from build123d import *

# Parameters (mm, degrees)
SKETCH1_R           = 34
SKETCH1_R_2         = 1.5
SKETCH1_R_3         = 6.8
SKETCH1_R_4         = 3.5
SKETCH1_W           = 3
SKETCH1_H           = 5
BOSS_EXTRUDE1_DEPTH = 5


with BuildPart() as part:
    # Sketch1 → Boss-Extrude1 (new body)
    with BuildSketch(Plane.XY):
        Circle(SKETCH1_R)
        with Locations((30, 0)):
            Circle(SKETCH1_R_2, mode=Mode.SUBTRACT)
        with Locations((-7.5, -12.990381057)):
            Circle(SKETCH1_R_2, mode=Mode.SUBTRACT)
        with Locations((-7.5, 12.990381057)):
            Circle(SKETCH1_R_2, mode=Mode.SUBTRACT)
        Circle(SKETCH1_R_3, mode=Mode.SUBTRACT)
        with Locations((-17.5, 20)):
            Circle(SKETCH1_R_4, mode=Mode.SUBTRACT)
        with Locations(Location((17.5, 20, 0), (0, 0, 180))):
            Circle(SKETCH1_R_4, mode=Mode.SUBTRACT)
        with Locations(Location((-17.5, -20, 0), (0, 0, 180))):
            Circle(SKETCH1_R_4, mode=Mode.SUBTRACT)
        with Locations((17.5, -20)):
            Circle(SKETCH1_R_4, mode=Mode.SUBTRACT)
        with Locations((20.845079102, 9.72022002)):
            Circle(SKETCH1_R_2, mode=Mode.SUBTRACT)
        with Locations((-20.845079102, 9.72022002)):
            Circle(SKETCH1_R_2, mode=Mode.SUBTRACT)
        with Locations((0, -23)):
            Circle(SKETCH1_R_2, mode=Mode.SUBTRACT)
        Polygon((15.679612774, 8.966590392), (11.148073839, 6.853499083), (12.415928624, 4.134575722), (16.947467559, 6.247667031), align=None, mode=Mode.SUBTRACT)
        Polygon((24.742690644, 13.192773009), (29.27422958, 15.305864318), (30.542084365, 12.586940957), (26.01054543, 10.473849648), align=None, mode=Mode.SUBTRACT)
        Polygon((-16.947467559, 6.247667031), (-12.415928624, 4.134575722), (-11.148073839, 6.853499083), (-15.679612774, 8.966590392), align=None, mode=Mode.SUBTRACT)
        Polygon((-26.01054543, 10.473849648), (-30.542084365, 12.586940957), (-29.27422958, 15.305864318), (-24.742690644, 13.192773009), align=None, mode=Mode.SUBTRACT)
        with Locations((0, -30.5)):
            Rectangle(SKETCH1_W, SKETCH1_H, mode=Mode.SUBTRACT)
        with Locations((0, -15.5)):
            Rectangle(SKETCH1_W, SKETCH1_H, mode=Mode.SUBTRACT)
    extrude(amount=BOSS_EXTRUDE1_DEPTH)


solid = part.part
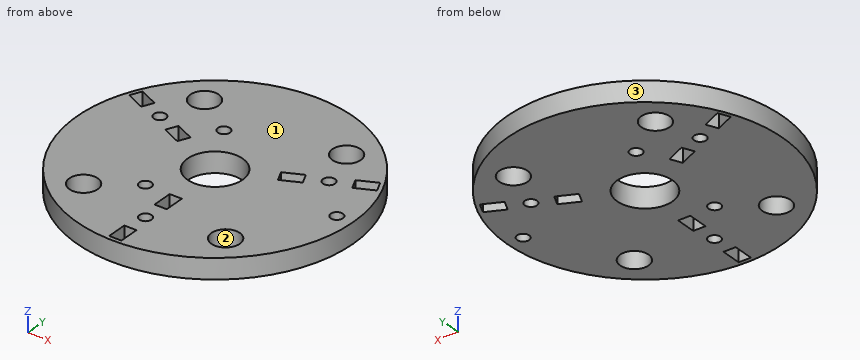
Source: CAD feature listing. Evaluate the final solid. Frame: model axes, mm. Face numbers are marked on the shaded views. Give positions to 0.01 mm unless a question says otherwise; leave off trailing zeros. Write each loop counter-clockwise with the first axis right and the second up, starting at its lowest first coordinate (ties: lowest second). Pieces come first, ordered by that corner, then holes. Notation, with made-up numbers: (-8, 19) -> (41, 19) arc R28 ccw to (41, 46) -> close; hole circle Ø1 at (65, 58). An arc over 180 degrees is marked (long way). Return JSON: item names as keys, results as strings. Group by question number.
1. Mould query, pull axis Y, two halves, no side actions, for the marked faces 1, 2 and 3. Classes: +Y half, -Y half, draft (parallel to the pull), parting line (faces both ways), or undercut.
2. Section D-D, the plane z = 3.85. Count the separate pieces of the cut face and the enclosed holes in it, then the cut area to 3 significant figures.
3. Section C-C, the plane x = 18.5. Output: boundary loops of the cut face in (y, z), then the cut area to 3 significant figures.
4. Section A-A, the plane x = 0. Output: boundary loops of the cut face in (y, z), then the cut area to 3 significant figures.
5. Material intervals for line 1 (X direction, y = 19, z = 2.75); line 2 (Y direction, x = -17.5, z = 1.7); line 3 (Y direction, x = -17, z = 1.2), sorted ascending. Write a range as from..to.
6. Section B-B, the plane y = -20. Output: boundary loops of the cut face in (x, z).
7. Pin query (flat end, axial travel): pin 1 Ø2.5 at (x, y) = (0, -23) entering from +Z; pin 2 Ø1 at (x, z) = (16.5, 4) entering from -Y; pin 3 Ø2.5 at (x, z) = (0.5, 2.5) entering from +Y; pin 4 Ø1 at (x, z) = (6, 4.5) entering from +Y. Return the tip coordinate at first contact, or that it passes through.
Determined:
{
 "1": {"face 1": "draft", "face 2": "undercut", "face 3": "parting line"},
 "2": {"separate pieces": "1", "enclosed holes": "17", "area": "3,200 mm2"},
 "3": {"outline": "(-28.53, 0) -> (-23.35, 0) -> (-23.35, 5) -> (-28.53, 5) -> close; (-16.65, 0) -> (16.65, 0) -> (16.65, 5) -> (-16.65, 5) -> close; (23.35, 0) -> (28.53, 0) -> (28.53, 5) -> (23.35, 5) -> close", "area": "218 mm2"},
 "4": {"outline": "(-34, 0) -> (-33, 0) -> (-33, 5) -> (-34, 5) -> close; (-28, 0) -> (-24.5, 0) -> (-24.5, 5) -> (-28, 5) -> close; (-21.5, 0) -> (-18, 0) -> (-18, 5) -> (-21.5, 5) -> close; (-13, 0) -> (-6.8, 0) -> (-6.8, 5) -> (-13, 5) -> close; (6.8, 0) -> (34, 0) -> (34, 5) -> (6.8, 5) -> close", "area": "207 mm2"},
 "5": {"line 1": "x = -28.2..-20.85, -14.15..14.15, 20.85..28.2", "line 2": "y = -29.15..-23.5, -16.5..16.5, 23.5..29.15", "line 3": "y = -29.44..-23.46, -16.54..16.54, 23.46..29.44"},
 "6": {"outline": "(-27.5, 0) -> (-21, 0) -> (-21, 5) -> (-27.5, 5) -> close; (-14, 0) -> (14, 0) -> (14, 5) -> (-14, 5) -> close; (21, 0) -> (27.5, 0) -> (27.5, 5) -> (21, 5) -> close"},
 "7": {"pin 1": "passes through", "pin 2": "stops at y = -30", "pin 3": "stops at y = 34", "pin 4": "stops at y = 33.55"}
}
